```python
from build123d import *

# Parameters (mm, degrees)
SKETCH2_W              = 38
SKETCH2_H              = 26
BOSS_EXTRUDE1_DEPTH    = 1.5875
CUT_EXTRUDE1_DEPTH     = 47.070816753
FILLET1_R              = 3.175
SKETCH6_R              = 1.55
CUT_EXTRUDE2_DEPTH     = 47.070816753
MOVE_FACE1_OUTLINE_R   = 1.55
MOVE_FACE1_OUTLINE_R_2 = 1.4738
MOVE_FACE1_DEPTH       = 1.5875


# Read off the part's stored shape, not the designer's step: Move Face1
with BuildPart() as part:
    # Sketch2 → Boss-Extrude1 (new body)
    with BuildSketch(Plane.XY):
        with Locations((19, 13)):
            Rectangle(SKETCH2_W, SKETCH2_H)
    extrude(amount=BOSS_EXTRUDE1_DEPTH)

    # Sketch3 → Cut-Extrude1 (cut, through all)
    with BuildSketch(Plane.XY.offset(1.5875)):
        Polygon((7.1, 21.1), (8.9, 21.1), (8.9, 24.2), (11.9, 24.2), (11.9, 21.1), (13.7, 21.1), (13.7, 4.9), (11.9, 4.9), (11.9, 1.8), (8.9, 1.8), (8.9, 4.9), (7.1, 4.9), align=None)
        Polygon((15.7, 21.1), (17.5, 21.1), (17.5, 24.2), (20.5, 24.2), (20.5, 21.1), (22.3, 21.1), (22.3, 4.9), (20.5, 4.9), (20.5, 1.8), (17.5, 1.8), (17.5, 4.9), (15.7, 4.9), align=None)
        Polygon((24.3, 21.1), (26.1, 21.1), (26.1, 24.2), (29.1, 24.2), (29.1, 21.1), (30.9, 21.1), (30.9, 4.9), (29.1, 4.9), (29.1, 1.8), (26.1, 1.8), (26.1, 4.9), (24.3, 4.9), align=None)
    extrude(amount=-CUT_EXTRUDE1_DEPTH, mode=Mode.SUBTRACT)

    # Fillet1
    fillet1_edges = [part.edges().sort_by_distance(p)[0] for p in [
        (0, 26, 0.79375),
        (38, 26, 0.79375),
        (38, 0, 0.79375),
        (0, 0, 0.79375),
    ]]
    fillet(fillet1_edges, radius=FILLET1_R)

    # Sketch6 → Cut-Extrude2 (cut, through all)
    with BuildSketch(Plane.XY.offset(1.5875)):
        with Locations((3.175, 22.825)):
            Circle(SKETCH6_R)
        with Locations((34.825, 22.825)):
            Circle(SKETCH6_R)
        with Locations((34.825, 3.175)):
            Circle(SKETCH6_R)
        with Locations((3.175, 3.175)):
            Circle(SKETCH6_R)
    extrude(amount=-CUT_EXTRUDE2_DEPTH, mode=Mode.SUBTRACT)

    # Move Face1 outline → Move Face1 (add)
    # profile 1 of 8: a face of its own
    with BuildSketch(Plane.XY):
        with BuildLine():
            Line((-0.0762, 22.825), (-0.0762, 3.175))
            ThreePointArc((-0.0762, 3.175), (0.876054433, 0.876054433), (3.175, -0.0762))
            Line((3.175, -0.0762), (34.825, -0.0762))
            ThreePointArc((34.825, -0.0762), (37.123945567, 0.876054433), (38.0762, 3.175))
            Line((38.0762, 3.175), (38.0762, 22.825))
            ThreePointArc((38.0762, 22.825), (37.123945567, 25.123945567), (34.825, 26.0762))
            Line((34.825, 26.0762), (3.175, 26.0762))
            ThreePointArc((3.175, 26.0762), (0.876054433, 25.123945567), (-0.0762, 22.825))
        make_face()
        with BuildLine():
            ThreePointArc((3.175, 0), (0.92993597, 0.92993597), (0, 3.175))
            Line((0, 3.175), (0, 22.825))
            ThreePointArc((0, 22.825), (0.92993597, 25.07006403), (3.175, 26))
            Line((3.175, 26), (34.825, 26))
            ThreePointArc((34.825, 26), (37.07006403, 25.07006403), (38, 22.825))
            Line((38, 22.825), (38, 3.175))
            ThreePointArc((38, 3.175), (37.07006403, 0.92993597), (34.825, 0))
            Line((34.825, 0), (3.175, 0))
        make_face(mode=Mode.SUBTRACT)
    # profile 2 of 8: a face of its own
    with BuildSketch(Plane.XY):
        Polygon((26.1, 21.1), (24.3, 21.1), (24.3, 4.9), (26.1, 4.9), (26.1, 1.8), (29.1, 1.8), (29.1, 4.9), (30.9, 4.9), (30.9, 21.1), (29.1, 21.1), (29.1, 24.2), (26.1, 24.2), align=None)
        Polygon((24.3762, 4.9762), (24.3762, 21.0238), (26.1762, 21.0238), (26.1762, 24.1238), (29.0238, 24.1238), (29.0238, 21.0238), (30.8238, 21.0238), (30.8238, 4.9762), (29.0238, 4.9762), (29.0238, 1.8762), (26.1762, 1.8762), (26.1762, 4.9762), align=None, mode=Mode.SUBTRACT)
    # profile 3 of 8: a face of its own
    with BuildSketch(Plane.XY):
        Polygon((17.5, 24.2), (17.5, 21.1), (15.7, 21.1), (15.7, 4.9), (17.5, 4.9), (17.5, 1.8), (20.5, 1.8), (20.5, 4.9), (22.3, 4.9), (22.3, 21.1), (20.5, 21.1), (20.5, 24.2), align=None)
        Polygon((15.7762, 21.0238), (17.5762, 21.0238), (17.5762, 24.1238), (20.4238, 24.1238), (20.4238, 21.0238), (22.2238, 21.0238), (22.2238, 4.9762), (20.4238, 4.9762), (20.4238, 1.8762), (17.5762, 1.8762), (17.5762, 4.9762), (15.7762, 4.9762), align=None, mode=Mode.SUBTRACT)
    # profile 4 of 8: a face of its own
    with BuildSketch(Plane.XY):
        Polygon((8.9, 24.2), (8.9, 21.1), (7.1, 21.1), (7.1, 4.9), (8.9, 4.9), (8.9, 1.8), (11.9, 1.8), (11.9, 4.9), (13.7, 4.9), (13.7, 21.1), (11.9, 21.1), (11.9, 24.2), align=None)
        Polygon((7.1762, 21.0238), (8.9762, 21.0238), (8.9762, 24.1238), (11.8238, 24.1238), (11.8238, 21.0238), (13.6238, 21.0238), (13.6238, 4.9762), (11.8238, 4.9762), (11.8238, 1.8762), (8.9762, 1.8762), (8.9762, 4.9762), (7.1762, 4.9762), align=None, mode=Mode.SUBTRACT)
    # profile 5 of 8: a face of its own
    with BuildSketch(Plane.XY):
        with Locations((3.175, 22.825)):
            Circle(MOVE_FACE1_OUTLINE_R)
        with Locations((3.175, 22.825)):
            Circle(MOVE_FACE1_OUTLINE_R_2, mode=Mode.SUBTRACT)
    # profile 6 of 8: a face of its own
    with BuildSketch(Plane.XY):
        with Locations((34.825, 22.825)):
            Circle(MOVE_FACE1_OUTLINE_R)
        with Locations((34.825, 22.825)):
            Circle(MOVE_FACE1_OUTLINE_R_2, mode=Mode.SUBTRACT)
    # profile 7 of 8: a face of its own
    with BuildSketch(Plane.XY):
        with Locations((34.825, 3.175)):
            Circle(MOVE_FACE1_OUTLINE_R)
        with Locations((34.825, 3.175)):
            Circle(MOVE_FACE1_OUTLINE_R_2, mode=Mode.SUBTRACT)
    # profile 8 of 8: a face of its own
    with BuildSketch(Plane.XY):
        with Locations((3.175, 3.175)):
            Circle(MOVE_FACE1_OUTLINE_R)
        with Locations((3.175, 3.175)):
            Circle(MOVE_FACE1_OUTLINE_R_2, mode=Mode.SUBTRACT)
    extrude(amount=MOVE_FACE1_DEPTH)


solid = part.part
```
Geometry check sheet. Reference: the model listing, model coordinates, mm. A direction names the side the tool comes from. Give positions to 0.01 mm unless a question says otherwise; leave off trailing zeros. Order: outer loops, then holes, each group sorted by start corner. A loop starts at its lowest first (then second) coordinate and runs counter-clockwise, first axis right, second up. Notation, with made-up numbers: (-36.75, 12) -> (-21.75, 12) arc R12 ccw to (-21.75, 33) -> close; hole circle Ø5 at (70, 58.25). An arc over 180 degrees is marked (long way). Write each question's results on one line, items separated by ' | '. Start each with the question number.
(1) Sectioned sample at B-B (y = 8.25). Enter the section's corners in (x, z), plus the area to 3 significant figures.
(2) Gauge pin test, flat end, axial feed: P1, Ø10, axis at x = 17, y = 7.5, coming from the -Z side. Record the tip position at first contact, or that the pin passes through.
(3) Sectioned sample at A-A (x = 10). Enter the section's corners in (y, z).
(4) Access from +Z, -Z, +X, -X, +Y, -Y to the whole of each face (thin tool, end or side, straight path). Record for faces 1 (the face through (25, 4.976, 1)), 2 (the face through (0.9, 25.15, 0.78)).
(5) Scan lines: line 1 (X direction, y = 5.5, z = 0.85); line 2 (Y direction, x = 21, z = 0.6); line 3 (X direction, y = 3.25, z = 0.85). Record each from-to range of solid material in increasing order.
(6) Sectioned sample at C-C (z = 0.7). Give the number of separate pieces and of enclosed holes in the cut face, plus the area to 3 significant figures.
Answer below:
1) outline: (-0.08, 0) -> (7.18, 0) -> (7.18, 1.59) -> (-0.08, 1.59) -> close; (13.62, 0) -> (15.78, 0) -> (15.78, 1.59) -> (13.62, 1.59) -> close; (22.22, 0) -> (24.38, 0) -> (24.38, 1.59) -> (22.22, 1.59) -> close; (30.82, 0) -> (38.08, 0) -> (38.08, 1.59) -> (30.82, 1.59) -> close | area: 29.9 mm2
2) P1: z = 0
3) outline: (-0.08, 0) -> (1.88, 0) -> (1.88, 1.59) -> (-0.08, 1.59) -> close; (24.12, 0) -> (26.08, 0) -> (26.08, 1.59) -> (24.12, 1.59) -> close
4) face 1: +Z, -Z | face 2: +Z, -Z, -X, +Y
5) line 1: -0.08 to 7.18, 13.62 to 15.78, 22.22 to 24.38, 30.82 to 38.08 | line 2: -0.08 to 4.98, 21.02 to 26.08 | line 3: -0.08 to 1.7, 4.65 to 8.98, 11.82 to 17.58, 20.42 to 26.18, 29.02 to 33.35, 36.3 to 38.08
6) separate pieces: 1 | enclosed holes: 7 | area: 598 mm2
